Part model, mm, in its own coordinate system. Round coordinates to 2 decimals unless told otherwise and drop trailing zeros. Write each loop counter-clockwise with the first axis right and the second up, starting at its lowest first coordinate (ties: lowest second). Pieces come first, ordered by that corner, then holes. Notation, with made-up numbers: M -28.5,38.25 L 8.5,38.25 A16 ccw 8.5,46.25 Z; hole C 89,-5.75 d2. An arc over 180 degrees is marked long. Use one line per item in the form item = value. Start each with the question number.
Item 1: Flat gauge pins, fed straight in: pin 1 Ø2 at (y, z) = (50.5, -126.5) entering from +X; pin 2 Ø10 at (x, z) = (40, -445.5) entering from -Y; pin 3 Ø10 at (x, z) = (5.5, -409.5) entering from +Y (3 decimals). Where does each tip first touch, or does it go through?
Item 2: Cut at B-B, the plane x = 50.5. Give the cut face in (y, z), then the cut area to 3 significant figures.
Item 3: Cut at C-C, the plane y = 61.5. Give the cut face in (x, z), then the cut area to 3 significant figures.
Item 4: Probe L1, parallel to X at y = 50.5, z = -380; L2, parallel to X at y = 5.5, z = -444.5; L3, parallel to Y at x = 4.5, z = -339 (3 decimals). List the from-to ranges inside material, lowest first.
from build123d import *

# Parameters (mm, degrees)
EXTRUDE_THIN1_DEPTH = 738.1875
FILLET1_R           = 1.651


with BuildPart() as part:
    # Sketch1 → Extrude-Thin1 (new body)
    with BuildSketch(Plane.XY):
        with BuildLine():
            Line((0, 0), (0, 22.225))
            Line((0, 22.225), (14.2875, 22.225))
            ThreePointArc((14.2875, 22.225), (31.125480227, 29.199519773), (38.1, 46.0375))
            Line((38.1, 46.0375), (38.1, 73.81875))
            Line((38.1, 73.81875), (57.15, 73.81875))
            Line((57.15, 73.81875), (57.15, 72.16775))
            Line((57.15, 72.16775), (39.751, 72.16775))
            Line((39.751, 72.16775), (39.751, 46.0375))
            ThreePointArc((39.751, 46.0375), (32.292913523, 28.032086477), (14.2875, 20.574))
            Line((14.2875, 20.574), (1.651, 20.574))
            Line((1.651, 20.574), (1.651, 0))
            Line((1.651, 0), (0, 0))
        make_face()
    extrude(amount=-EXTRUDE_THIN1_DEPTH)

    # Fillet1
    fillet1_edges = [part.edges().sort_by_distance(p)[0] for p in [
        (0, 22.225, -369.09375),
        (38.1, 73.81875, -369.09375),
    ]]
    fillet(fillet1_edges, radius=FILLET1_R)


solid = part.part
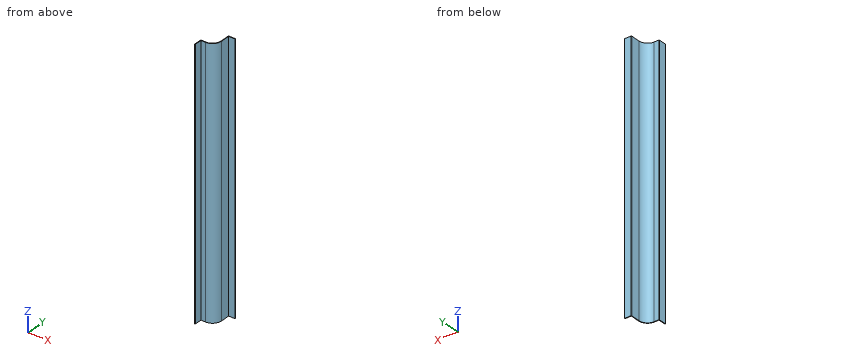
Model answer:
q1.pin_1 = 39.75
q1.pin_2 = 31.23
q1.pin_3 = 22.225
q2.outline = M 72.17,-738.19 L 73.82,-738.19 L 73.82,0 L 72.17,0 Z
q2.area = 1,220 mm²
q3.outline = M 38.1,-738.19 L 39.75,-738.19 L 39.75,0 L 38.1,0 Z
q3.area = 1,220 mm²
q4.L1 = 38.1 to 39.75
q4.L2 = 0 to 1.65
q4.L3 = 20.574 to 22.225
